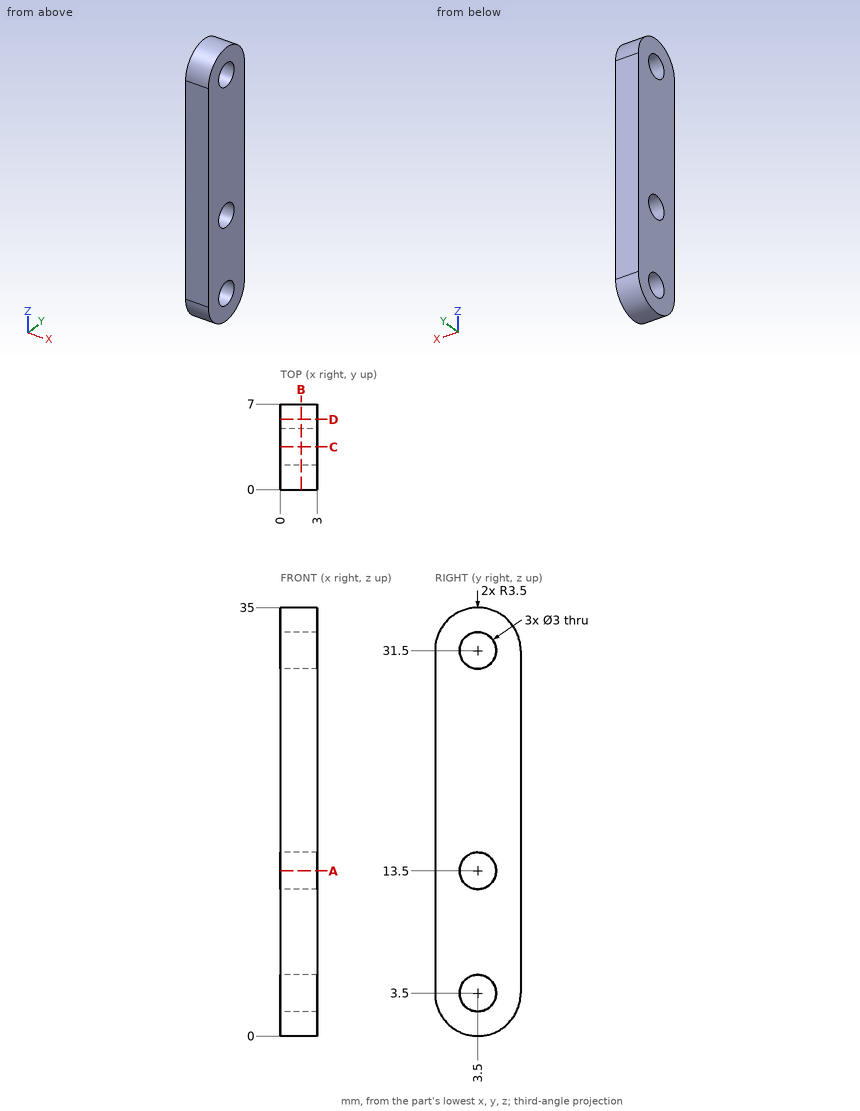
Can you work these out from the drawing? Everything is in mm from the part's minimum corner. Coordinates: 2 decimals unless noted, no trailing zeros. Write each loop counter-clockwise with the first axis right and the second up, starting at its lowest first coordinate (ties: lowest second). Pieces come first, ordered by that corner, then holes. Notation, with made-up numbers: (-20, -2.5) -> (12, -2.5) arc R8 cw to (12, 6.5) -> close; hole circle Ø7 at (32.5, -18.5). An arc over 180 degrees is marked (long way). Write item = value, one per line.
(1) Imagine slicing it at A-A (z = 13.5). Please give me the cut outline in (x, y), and give its area (3 significant figures).
Verdict:
outline = (0, 0) -> (3, 0) -> (3, 2) -> (0, 2) -> close; (0, 5) -> (3, 5) -> (3, 7) -> (0, 7) -> close
area = 12.0 mm^2
(2) Imagine slicing it at B-B (x = 1.7). Please give me the cut outline in (y, z).
Verdict:
outline = (0, 3.5) arc R3.5 ccw to (7, 3.5) -> (7, 31.5) arc R3.5 ccw to (0, 31.5) -> close; hole circle Ø3 at (3.5, 3.5); hole circle Ø3 at (3.5, 13.5); hole circle Ø3 at (3.5, 31.5)
(3) For pin 1 (1.5 mm diameter, centred on x = 2, y = 5, fed in from -Z); pin 2 (2.5 mm diameter, centred on y = 3.5, z = 13.5, fed in from -X), each with a flat end and sliding along its axis, tell me the tip position at first contact or that it passes through.
Verdict:
pin_1 = 0.08
pin_2 = through
(4) Imagine slicing it at C-C (y = 3.5). Please give me the cut outline in (x, z).
Verdict:
outline = (0, 0) -> (3, 0) -> (3, 2) -> (0, 2) -> close; (0, 5) -> (3, 5) -> (3, 12) -> (0, 12) -> close; (0, 15) -> (3, 15) -> (3, 30) -> (0, 30) -> close; (0, 33) -> (3, 33) -> (3, 35) -> (0, 35) -> close
(5) If I drill on probe 1 along Z at (x, y) = (1.05, 3.5); probe 2 along Y at (x, z) = (1.7, 13.5); probe 3 along Z at (x, y) = (1, 3), over which ranges is the centre line in solid material (lowest first)?
Verdict:
probe_1 = 0 to 2, 5 to 12, 15 to 30, 33 to 35
probe_2 = 0 to 2, 5 to 7
probe_3 = 0.04 to 2.09, 4.91 to 12.09, 14.91 to 30.09, 32.91 to 34.96
(6) Imagine slicing it at D-D (y = 5.75). Please give me the cut outline in (x, z).
Verdict:
outline = (0, 0.82) -> (3, 0.82) -> (3, 34.18) -> (0, 34.18) -> close
